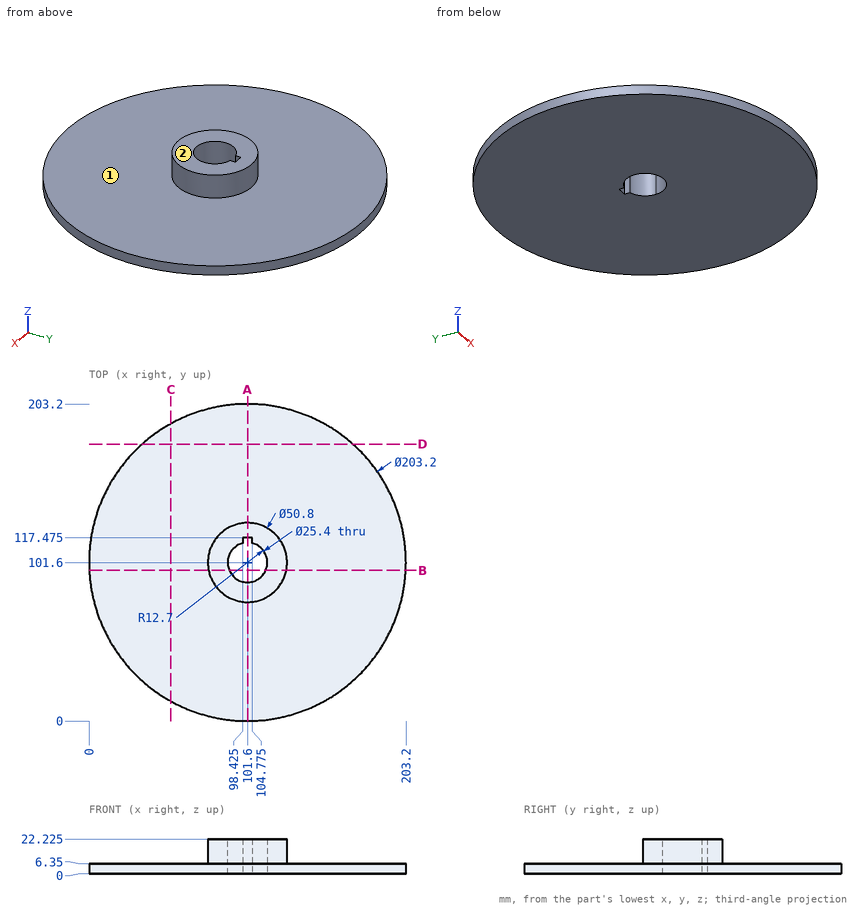
Drawing for the job (mm, zero at the part's lowest x, y, z). A direction names the side the tool comes from. Coordinates: 2 decimals unless noted, no trailing zeros. Write each loop counter-clockwise with the first axis right and the second up, starting at its lowest first coordinate (ties: lowest second). Pieces come first, ordered by that corner, then holes. Notation, with made-up numbers: (78.5, -0.5) -> (118.5, -0.5) arc R28 cw to (118.5, 34.5) -> close; hole circle Ø5 at (19, 39). An arc over 180 degrees is marked (long way). One line per item, written item: value. Start each with the question number.
1) Flat gauge pins, fed straight in: pin 1 Ø3 at (y, z) = (115.5, 6) entering from -X; pin 2 Ø8 at (x, y) = (151.5, 63.5) entering from +Z; pin 3 Ø4 at (y, z) = (115, 6) entering from +X; pin 4 Ø6 at (y, z) = (58, 9.5) entering from -X. Where does each tip first touch, or does it go through?
2) Slice it at D-D on y = 177.5. Write the cut outline in (x, z), then the cut area to 3 significant figures.
3) Slice it at B-B on y = 96.5. Write the cut outline in (x, z) (3 decimals), then the cut area to 3 significant figures.
4) Which spindle directions (+Z, -Z, +X, -X, +Y, -Y) get a long thin tool onto all of the face, cutting with end or side? Do the marked faces 1 and 2. Say none if no direction does.
5) Slice it at C-C on x = 52.5. Write the cut outline in (y, z).
6) Probe probe 1 along Y at (x, z) = (101.6, 16) (3 decimals); probe 2 along Z at (x, y) = (55.5, 168.5); probe 3 along Y at (x, z) = (108.5, 12.75). List the from-to ranges inside material, lowest first.
7) Slice it at A-A on x = 101.6. Write the cut outline in (y, z) (3 decimals), then the cut area to 3 significant figures.
Answers follow:
1. pin 1: x = 0.76
1. pin 2: z = 6.35
1. pin 3: x = 202.56
1. pin 4: through
2. outline: (34.06, 0) -> (169.14, 0) -> (169.14, 6.35) -> (34.06, 6.35) -> close
2. area: 858 mm2
3. outline: (0.128, 0) -> (89.969, 0) -> (89.969, 22.225) -> (76.717, 22.225) -> (76.717, 6.35) -> (0.128, 6.35) -> close; (113.231, 0) -> (203.072, 0) -> (203.072, 6.35) -> (126.483, 6.35) -> (126.483, 22.225) -> (113.231, 22.225) -> close
3. area: 1,560 mm2
4. face 1: +Z
4. face 2: +Z, +X, -X, +Y, -Y
5. outline: (12.65, 0) -> (190.55, 0) -> (190.55, 6.35) -> (12.65, 6.35) -> close
6. probe 1: 76.2 to 88.9, 117.475 to 127
6. probe 2: 0 to 6.35
6. probe 3: 77.16 to 90.94, 112.26 to 126.04
7. outline: (0, 0) -> (88.9, 0) -> (88.9, 22.225) -> (76.2, 22.225) -> (76.2, 6.35) -> (0, 6.35) -> close; (117.475, 0) -> (203.2, 0) -> (203.2, 6.35) -> (127, 6.35) -> (127, 22.225) -> (117.475, 22.225) -> close
7. area: 1,460 mm2
